from build123d import *

# Parameters (mm, degrees)
F0_W     = 10.16
F0_H     = 10.16
F0_W_2   = 27.94
F1_DEPTH = 10.16
F2_D     = 4.4958
F3_D     = 4.4958
F4_D     = 4.4958
F5_D     = 4.4958
F7_D     = 4.4958
F10_D    = 4.4958
F11_D    = 4.4958


# Not quite as in the source:
# - a feature names something its author has since deleted; it is built from what else it names


with BuildPart() as f1:
    # F0 (on Top) → F1 (new body)
    with BuildSketch(Plane.XY):
        Polygon((-19.05, 32.0548), (-19.05, -5.08), (-8.89, -5.08), (-8.89, 5.08), (-8.89, 21.8948), (-8.89, 32.0548), align=None)
        with Locations((-13.97, -10.16)):
            Rectangle(F0_W, F0_H)
        with Locations((5.08, 0)):
            Rectangle(F0_W_2, F0_H)
        with Locations((-13.97, 37.1348)):
            Rectangle(F0_W, F0_H)
        with Locations((5.08, 26.9748)):
            Rectangle(F0_W_2, F0_H)
    extrude(amount=F1_DEPTH)

    # F2 (through all)
    with Locations(Plane(origin=(0, 0, 0), x_dir=(1, 0, 0), z_dir=(0, 0, -1))):
        with Locations((13.4874, 0)):
            Hole(F2_D / 2)

    # F3 (through all)
    with Locations(Plane(origin=(0, 0, 0), x_dir=(1, 0, 0), z_dir=(0, 0, -1))):
        with Locations((-13.4874, 0)):
            Hole(F3_D / 2)

    # F4 (through all)
    with Locations(Plane(origin=(0, 0, 0), x_dir=(1, 0, 0), z_dir=(0, 0, -1))):
        with Locations((-13.4874, -26.9748)):
            Hole(F4_D / 2)

    # F5 (through all)
    with Locations(Plane(origin=(0, 0, 0), x_dir=(1, 0, 0), z_dir=(0, 0, -1))):
        with Locations((13.4874, -26.9748)):
            Hole(F5_D / 2)

    # F7 (through all)
    with Locations(Plane.YZ.offset(-8.89)):
        with Locations((13.4874, 5.08)):
            Hole(F7_D / 2)

    # F10 (through all)
    with Locations(Plane.YZ.offset(-8.89)):
        with Locations((-10.16, 5.08)):
            Hole(F10_D / 2)

    # F11 (through all)
    with Locations(Plane.YZ.offset(-8.89)):
        with Locations((37.1348, 5.08)):
            Hole(F11_D / 2)


solid = f1.part
Read the model definition and answer for the solid it produces. Units are mm, in the model's axes. A direction names the side the tool comes from. Give positions to 0.01 mm unless a question says otherwise; leave off trailing zeros. Write each loop counter-clockwise with the first axis right and the second up, starting at its lowest first coordinate (ties: lowest second). Pieces come first, ordered by that corner, then holes. Notation, with made-up numbers: (63, 65) - (116, 65) arc R27 cw to (116, 93) - close; hole circle Ø9 at (-13.5, -4). An arc over 180 degrees is marked (long way). Use CSV: the item, a comma, the result in double quotes. Start each with the question number.
(1) Find section A-A (x = 10). Give the vertices of the cut face in (y, z).
(2) Find section C-C (y = 0). Give the vertices of the cut face in (x, z).
(3) Find section B-B (y = -10.16). Give the vertices of the cut face in (x, z), plus the area to 3 significant figures.
(4) Consider line 1 along Y through (x, z) = (-16.5, 5.25); line 2 along X through (y, z) = (-1.5, 6); line 3 along Y through (x, z) = (2.5, 6.25). Determine where each line is inside the solid, lowest interval first.
(5) For faces 1 (the flat face through (5, 5.08, 5)), 2 (the flat face through (5, -5.08, 5)), 3 (the flat face through (5, 32.055, 5)), determine the directions among +Z, -Z, +X, -X, +Y, -Y from which every point of the face is accessible in a straight line to the end or side of a thin tool.
(6) Find section D-D (z = 4). Give the vertices of the cut face in (x, y), plus the area to 3 significant figures.
(7) Determine the mould class of faces 4 (the flat face through (-10, 11, 10.16)), 5 (the cylindrical face through (-14.041, 38.919, 3.712)), 6 (the flat face through (-14, -15.24, 5)), 7 (the flat face through (5, 21.895, 5)) for opening direction Y: +Y half, -Y half, draft (parallel to the pull), parting line (faces both ways), or undercut.
(8) Given P1, Ø5, axis at y = -10.5, z = 2.5, coming from the +X side; P2, Ø5, axis at x = 8.5, z = 5.5, coming from the +Y side; P3, Ø5, axis at x = 7.5, z = 3, coming from the -Y side, each flat-ended and moving along its own axis, determine where each tip first touches the part or whether it passes through.
Findings below:
1,outline,"(-5.08, 0) - (5.08, 0) - (5.08, 10.16) - (-5.08, 10.16) - close; (21.89, 0) - (32.05, 0) - (32.05, 10.16) - (21.89, 10.16) - close"
2,outline,"(-19.05, 0) - (-15.74, 0) - (-15.74, 10.16) - (-19.05, 10.16) - close; (-11.24, 0) - (11.24, 0) - (11.24, 10.16) - (-11.24, 10.16) - close; (15.74, 0) - (19.05, 0) - (19.05, 10.16) - (15.74, 10.16) - close"
3,outline,"(-19.05, 0) - (-8.89, 0) - (-8.89, 2.83) - (-19.05, 2.83) - close; (-19.05, 7.33) - (-8.89, 7.33) - (-8.89, 10.16) - (-19.05, 10.16) - close"
3,area,"57.5 mm2"
4,line 1,"-15.24 to -12.4, -7.92 to 11.25, 15.73 to 34.89, 39.38 to 42.21"
4,line 2,"-19.05 to -15.16, -11.81 to 11.81, 15.16 to 19.05"
4,line 3,"-5.08 to 5.08, 21.89 to 32.05"
5,face 1,"+Z, -Z, +X"
5,face 2,"+Z, -Z, +X, -Y"
5,face 3,"+Z, -Z, +X, +Y"
6,outline,"(-19.05, -15.24) - (-8.89, -15.24) - (-8.89, -12.13) - (-19.05, -12.13) - close; (-19.05, -8.19) - (-8.89, -8.19) - (-8.89, -5.08) - (19.05, -5.08) - (19.05, 5.08) - (-8.89, 5.08) - (-8.89, 11.52) - (-19.05, 11.52) - close; (-19.05, 15.46) - (-8.89, 15.46) - (-8.89, 21.89) - (19.05, 21.89) - (19.05, 32.05) - (-8.89, 32.05) - (-8.89, 35.16) - (-19.05, 35.16) - close; (-19.05, 39.11) - (-8.89, 39.11) - (-8.89, 42.21) - (-19.05, 42.21) - close; hole circle Ø4.5 at (-13.49, 0); hole circle Ø4.5 at (-13.49, 26.97); hole circle Ø4.5 at (13.49, 0); hole circle Ø4.5 at (13.49, 26.97)"
6,area,"968 mm2"
7,face 4,"draft"
7,face 5,"undercut"
7,face 6,"-Y half"
7,face 7,"undercut"
8,P1,"x = -8.89"
8,P2,"y = 32.05"
8,P3,"y = -5.08"
